```python
from build123d import *

# Parameters (mm, degrees)
BASE_DEPTH        = 3
BASE_DEPTH_BACK   = 7
SKETCH1_R         = 10
SKETCH2_R         = 1.5
HOLE1_DEPTH       = 19.934353276
HOLE1MIRROR_COUNT = 2
SKETCH3_R         = 1.5
HOLE2_DEPTH       = 19.445737601
HOLE2MIRROR_COUNT = 2
SKETCH4_R         = 1.5
HOLE3_DEPTH       = 19.389503466
HOLE3MIRROR_COUNT = 2
FILLET1_R         = 5


with BuildPart() as part:
    # Sketch1 → base (new, two sides: drawn at the far end of the back side and taken through both)
    with BuildSketch(Plane(origin=(0, 0, 0), x_dir=(1, 0, 0), z_dir=(0, 1, 0)).offset(-BASE_DEPTH_BACK)):
        with Locations(Location((0, 0, 0), (0, 0, 270))):
            Circle(SKETCH1_R)
    extrude(amount=BASE_DEPTH + BASE_DEPTH_BACK)

    # Sketch2 → hole1 (cut, through all)
    with BuildSketch(Plane(origin=(2.670502563, -1.093066116, 2.770130417), x_dir=(-0.6558691872850446, 0.22429081675253856, 0.7207837669443827), z_dir=(-0.6676256406563905, 0.27326652891267483, -0.692532604369038))):
        with Locations(Location((0, 0, 0), (0, 0, 346.516491398))):
            Circle(SKETCH2_R)
    hole1 = extrude(amount=-HOLE1_DEPTH, mode=Mode.SUBTRACT)

    # hole1mirror: hole1 ×2 about axis
    hole1mirror_axis = Axis((0, 5.5, 0), (0, -1, 0))
    for i in range(1, HOLE1MIRROR_COUNT):
        add(hole1.rotate(hole1mirror_axis, i * 360 / HOLE1MIRROR_COUNT), mode=Mode.SUBTRACT)

    # Sketch3 → hole2 (cut, through all)
    with BuildSketch(Plane(origin=(-0.941672921, -1.236067977, 3.685836142), x_dir=(-0.9718935871364875, 0.07382318789513377, -0.22354639834264944), z_dir=(0.23541823021467095, 0.3090169943749464, -0.921459035481267))):
        with Locations(Location((0, 0, 0), (0, 0, 90.062171088))):
            Circle(SKETCH3_R)
    hole2 = extrude(amount=-HOLE2_DEPTH, mode=Mode.SUBTRACT)

    # hole2mirror: hole2 ×2 about axis
    hole2mirror_axis = Axis((0, 5.5, 0), (0, -1, 0))
    for i in range(1, HOLE2MIRROR_COUNT):
        add(hole2.rotate(hole2mirror_axis, i * 360 / HOLE2MIRROR_COUNT), mode=Mode.SUBTRACT)

    # Sketch4 → hole3 (cut, through all)
    with BuildSketch(Plane(origin=(-3.717841, -1.236067977, 0.806098168), x_dir=(-0.19123247894507908, -0.06357892752956036, -0.979483465389136), z_dir=(0.9294602499075393, 0.30901699437494623, -0.20152454200243008))):
        with Locations(Location((0, 0, 0), (0, 0, 90))):
            Circle(SKETCH4_R)
    hole3 = extrude(amount=-HOLE3_DEPTH, mode=Mode.SUBTRACT)

    # hole3mirror: hole3 ×2 about axis
    hole3mirror_axis = Axis((0, 5.5, 0), (0, -1, 0))
    for i in range(1, HOLE3MIRROR_COUNT):
        add(hole3.rotate(hole3mirror_axis, i * 360 / HOLE3MIRROR_COUNT), mode=Mode.SUBTRACT)

    # Fillet1
    # the kernel refuses this fillet: 5 mm, written as the material it takes off along each edge
    with BuildSketch(Plane(origin=(0, -7, 0), x_dir=(0, 0, 1), z_dir=(-1, 0, 0))) as fillet1_piece_1:
        with BuildLine():
            CenterArc((10 - FILLET1_R, FILLET1_R), FILLET1_R, 270, 90)
            Line((10 - FILLET1_R, 0), (10, 0))
            Line((10, 0), (10, FILLET1_R))
        make_face()
    revolve(axis=Axis((0, -7, 0), (0, 1, 0)), mode=Mode.SUBTRACT)
    with BuildSketch(Plane(origin=(0, 3, 0), x_dir=(0, 0, 1), z_dir=(-1, 0, 0))) as fillet1_piece_2:
        with BuildLine():
            CenterArc((10 - FILLET1_R, -FILLET1_R), FILLET1_R, 0, 90)
            Line((10 - FILLET1_R, 0), (10, 0))
            Line((10, 0), (10, -FILLET1_R))
        make_face()
    revolve(axis=Axis((0, 3, 0), (0, 1, 0)), mode=Mode.SUBTRACT)


solid = part.part
```
Check sheet for the modelled part. Datum: model origin and axes. Units: mm. A direction names the side the tool comes from. Round coordinates to 2 decimals unless told otherwise and drop trailing zeros. Answer as CSV lines item,"result". Start each with the question number.
1) Draft check along X on faces 1 (the face through (0, 3, 0)), 2 (the face through (-6.05, -3.18, 2.42)). Enter one of: +X half, -X half, draft (parallel to the pull), parting line (faces both ways), or undercut.
2) Tool access check on faces 3 (the face through (0, -7, 0)), 4 (the face through (-3.7, -1.3, 0.8)). Record the directions out of +Z, -Z, +X, -X, +Y, -Y that give a thin tool (end or side, any length) a straight path to the whole face; none if there is none.
3) Scan lines: probe 1 along Y at (x, z) = (-3, 8); probe 2 along Z at (x, y) = (-6, -0.75); probe 3 along Z at (x, y) = (5.75, -5.25). Record each from-to range of solid material in increasing order.
4) Section check A-A (y = -0.5). Give the number of separate pieces and of enclosed holes in the cut face, then the cut area to 3 significant figures.
5) Depth check by flat-ended pin: pin 1 (1 mm diameter, centred on y = -4, z = 8, fed in from -X); pin 2 (5 mm diameter, centred on x = 2.5, y = -0.5, fed in from -Z); pin 3 (1 mm diameter, centred on y = 0, z = 4.5, fed in from +X). Enter the tip coordinate at first touch or a pass-through.
Determined:
1,face 1,"draft"
1,face 2,"undercut"
2,face 3,"+Z, -Z, +X, -X, -Y"
2,face 4,"none"
3,probe 1,"-5.53 to -4, -1.52 to 1.53"
3,probe 2,"-7.8 to 0.28, 2.16 to 7.8"
3,probe 3,"-6.66 to 6.66"
4,separate pieces,"1"
4,enclosed holes,"6"
4,area,"270 mm^2"
5,pin 1,"x = -6.04"
5,pin 2,"z = -9.99"
5,pin 3,"x = 8.79"
